The listing builds one solid part. Answer for the finished solid, in the listing's coordinates (mm). Coordinates: 2 decimals unless noted, no trailing zeros. Write each loop counter-clockwise with the first axis right and the second up, starting at its lowest first coordinate (ties: lowest second). Pieces come first, ordered by that corner, then holes.
(1) Given P1, Ø1, axis at y = -2.5, z = 7.5, coming from the -X side; P2, Ø2, axis at y = 0.5, z = 7.5, coming from the -X side; P3, Ø4, axis at x = -0.5, y = 2.5, coming from the -Z side; P4, Ø4, axis at y = -0.5, z = 3, coming from the +X side, each flat-ended and moving along its own axis, determine where each tip first touches the part or whether it passes through.
(2) The part is cut by section D-D on y = 1.5. Determine the outline of the cut face in (x, z).
(3) The part is cut by section B-B on y = -0.5. Determine the outline of the cut face in (x, z), plus the area to 3 significant figures.
(4) The part is cut by section A-A on z = 7.5. Determine the outline of the cut face in (x, y).
(5) For a pull along Y with two mould halves and no side action, classify faces 1 (the cylindrical face through (0, 0, 8)), 2 (the flat face through (0, 6.3, 4)), 3 (the flat face through (6.1, -0.09, 4.31)) as +Y half, -Y half, draft (parallel to the pull), parting line (faces both ways), or undercut.
(6) The part is cut by section C-C on x = 0.75. Determine the outline of the cut face in (y, z), plus the area to 3 significant figures.
(7) Straight lines are drawn through the part: line 1 (Y direction, x = 3.25, z = 7); line 2 (Z direction, x = 0.5, y = 0); line 3 (Y direction, x = 4.25, z = 7.5). For each, find the intervals that lie inside material, in ascending order.
from build123d import *

# Parameters (mm, degrees)
F3_DEPTH = 6.3
F2_R     = 1
F4_DEPTH = 15.501


with BuildPart() as f3:
    # F0 (on Front) → F3 (new body, symmetric)
    with BuildSketch(Plane.XZ):
        Polygon((-4.5, 0), (0, 0), (4.5, 0), (7.75, 8.75), (0, 8.75), (-7.75, 8.75), align=None)
    extrude(amount=F3_DEPTH, both=True)

    # F2 (on plane+point) → F4 (cut, through all)
    with BuildSketch(Plane.YZ.offset(7.75)):
        with Locations((0, 7)):
            Circle(F2_R)
    extrude(amount=-F4_DEPTH, mode=Mode.SUBTRACT)


solid = f3.part
Model answer:
1. P1: stops at x = -7.47
1. P2: stops at x = -7.66
1. P3: stops at z = 0
1. P4: stops at x = 6.36
2. outline: (-7.75, 8.75) - (-4.5, 0) - (4.5, 0) - (7.75, 8.75) - close
3. outline: (-7.75, 8.75) - (-7.42, 7.87) - (7.42, 7.87) - (7.75, 8.75) - close; (-6.78, 6.13) - (-4.5, 0) - (4.5, 0) - (6.78, 6.13) - close
3. area: 82.6 mm2
4. outline: (-7.29, -6.3) - (7.29, -6.3) - (7.29, -0.87) - (-7.29, -0.87) - close; (-7.29, 0.87) - (7.29, 0.87) - (7.29, 6.3) - (-7.29, 6.3) - close
5. face 1: undercut
5. face 2: +Y half
5. face 3: draft
6. outline: (-6.3, 0) - (6.3, 0) - (6.3, 8.75) - (-6.3, 8.75) - close; hole circle Ø2 at (0, 7)
6. area: 107 mm2
7. line 1: y = -6.3 to -1, 1 to 6.3
7. line 2: z = 0 to 6, 8 to 8.75
7. line 3: y = -6.3 to -0.87, 0.87 to 6.3
